from build123d import *

# Parameters (mm, degrees)
F0_W     = 25.4
F0_H     = 50.8
F0_W_2   = 22.225
F0_H_2   = 47.625
F1_DEPTH = 279.4
F2_R     = 2.5527
F3_DEPTH = 50.801
F4_R     = 2.5527
F5_DEPTH = 25.401


with BuildPart() as f1:
    # F0 (on Top) → F1 (new body)
    with BuildSketch(Plane.XY):
        Rectangle(F0_W, F0_H)
        Rectangle(F0_W_2, F0_H_2, mode=Mode.SUBTRACT)
    extrude(amount=F1_DEPTH)

    # F2 (on face) → F3 (cut, through all)
    with BuildSketch(Plane.XZ.offset(25.4)):
        with Locations((0, 266.7)):
            Circle(F2_R)
        with Locations((0, 241.3)):
            Circle(F2_R)
        with Locations((0, 215.9)):
            Circle(F2_R)
        with Locations((0, 190.5)):
            Circle(F2_R)
        with Locations((0, 165.1)):
            Circle(F2_R)
        with Locations((0, 139.7)):
            Circle(F2_R)
        with Locations((0, 114.3)):
            Circle(F2_R)
        with Locations((0, 88.9)):
            Circle(F2_R)
        with Locations((0, 63.5)):
            Circle(F2_R)
        with Locations((0, 38.1)):
            Circle(F2_R)
        with Locations((0, 12.7)):
            Circle(F2_R)
    extrude(amount=-F3_DEPTH, mode=Mode.SUBTRACT)

    # F4 (on face) → F5 (cut, through all)
    with BuildSketch(Plane(origin=(-12.7, 0, 0), x_dir=(0, -1, 0), z_dir=(-1, 0, 0))):
        with Locations((-12.7, 12.7)):
            Circle(F4_R)
        with Locations((12.7, 12.7)):
            Circle(F4_R)
        with Locations((-12.7, 38.1)):
            Circle(F4_R)
        with Locations((-12.7, 63.5)):
            Circle(F4_R)
        with Locations((-12.7, 88.9)):
            Circle(F4_R)
        with Locations((-12.7, 114.3)):
            Circle(F4_R)
        with Locations((-12.7, 139.7)):
            Circle(F4_R)
        with Locations((-12.7, 165.1)):
            Circle(F4_R)
        with Locations((-12.7, 190.5)):
            Circle(F4_R)
        with Locations((-12.7, 215.9)):
            Circle(F4_R)
        with Locations((-12.7, 241.3)):
            Circle(F4_R)
        with Locations((-12.7, 266.7)):
            Circle(F4_R)
        with Locations((12.7, 38.1)):
            Circle(F4_R)
        with Locations((12.7, 63.5)):
            Circle(F4_R)
        with Locations((12.7, 88.9)):
            Circle(F4_R)
        with Locations((12.7, 114.3)):
            Circle(F4_R)
        with Locations((12.7, 139.7)):
            Circle(F4_R)
        with Locations((12.7, 165.1)):
            Circle(F4_R)
        with Locations((12.7, 190.5)):
            Circle(F4_R)
        with Locations((12.7, 215.9)):
            Circle(F4_R)
        with Locations((12.7, 241.3)):
            Circle(F4_R)
        with Locations((12.7, 266.7)):
            Circle(F4_R)
    extrude(amount=-F5_DEPTH, mode=Mode.SUBTRACT)


solid = f1.part
Work out the finished part from the listing and answer in its coordinate system (mm). Coordinates: 2 decimals unless noted, no trailing zeros. Write each loop counter-clockwise with the first axis right and the second up, starting at its lowest first coordinate (ties: lowest second). Pieces come first, ordered by that corner, then holes.
1. The part is cut by section D-D, the plane z = 204. Write down the section's boundary in (x, y).
Results list:
outline: (-12.7, -25.4) - (12.7, -25.4) - (12.7, 25.4) - (-12.7, 25.4) - close; hole (-11.11, -23.81) - (11.11, -23.81) - (11.11, 23.81) - (-11.11, 23.81) - close
2. The part is cut by section B-B, the plane x = 6.25. Write down the section's boundary in (y, z), and give its area (3 significant figures).
Results list:
outline: (-25.4, 0) - (-23.81, 0) - (-23.81, 279.4) - (-25.4, 279.4) - close; (23.81, 0) - (25.4, 0) - (25.4, 279.4) - (23.81, 279.4) - close
area: 887 mm2
3. Consider line 1 along Y through (x, z) = (12.2, 190.5); line 2 along X through (y, z) = (22, 110.5); line 3 along Y through (x, z) = (-5.75, 224). Determine where each line is inside the solid, lowest interval first.
Results list:
line 1: y = -25.4 to -15.25, -10.15 to 10.15, 15.25 to 25.4
line 2: x = -12.7 to -11.11, 11.11 to 12.7
line 3: y = -25.4 to -23.81, 23.81 to 25.4
4. The part is cut by section C-C, the plane y = -2. Write down the section's boundary in (x, z), and give its area (3 significant figures).
Results list:
outline: (-12.7, 0) - (-11.11, 0) - (-11.11, 279.4) - (-12.7, 279.4) - close; (11.11, 0) - (12.7, 0) - (12.7, 279.4) - (11.11, 279.4) - close
area: 887 mm2
5. The part is cut by section A-A, the plane z = 114.3. State how many separate pieces and enclosed holes the cut face has, and give its area (3 significant figures).
Results list:
separate pieces: 6
enclosed holes: 0
area: 183 mm2
6. A flat-ended cylindrical pin translates along its axis: pin 1 (6.5 mm diameter, centred on y = 12.7, z = 63.5, fed in from +X). Find the tip coordinate at first contact, or state that the pin passes through.
Results list:
pin 1: stops at x = 12.7
